The listing builds one solid part. Answer for the finished solid, in the listing's coordinates (mm). Face numbers are marked on the shaded views. Coordinates: 2 decimals unless noted, no trailing zeros. Order: outer loops, then holes, each group sorted by start corner. A loop starts at its lowest first (then second) coordinate and runs counter-clockwise, first axis right, second up.
from build123d import *

# Parameters (mm, degrees)
IZIM1_R                     = 8
IZIM1_R_2                   = 7
Y_KSEKLIK_EKSTR_ZYON1_DEPTH = 180
IZIM2_R                     = 1.5
KES_EKSTR_ZYON1_DEPTH       = 10


with BuildPart() as part:
    # Çizim1 → Yükseklik-Ekstrüzyon1 (new body)
    with BuildSketch(Plane(origin=(0, 0, 0), x_dir=(1, 0, 0), z_dir=(0, 1, 0))):
        with Locations(Location((0, 0, 0), (0, 0, 90))):
            Circle(IZIM1_R)
        with Locations(Location((0, 0, 0), (0, 0, 90))):
            Circle(IZIM1_R_2, mode=Mode.SUBTRACT)
    extrude(amount=Y_KSEKLIK_EKSTR_ZYON1_DEPTH)

    # Çizim2 → Kes-Ekstrüzyon1 (cut, symmetric)
    with BuildSketch(Plane.XY):
        with Locations((0, 11)):
            Circle(IZIM2_R)
        with Locations((0, 168)):
            Circle(IZIM2_R)
        with Locations((0, 158)):
            Circle(IZIM2_R)
        with Locations((0, 21)):
            Circle(IZIM2_R)
    extrude(amount=KES_EKSTR_ZYON1_DEPTH, both=True, mode=Mode.SUBTRACT)


solid = part.part
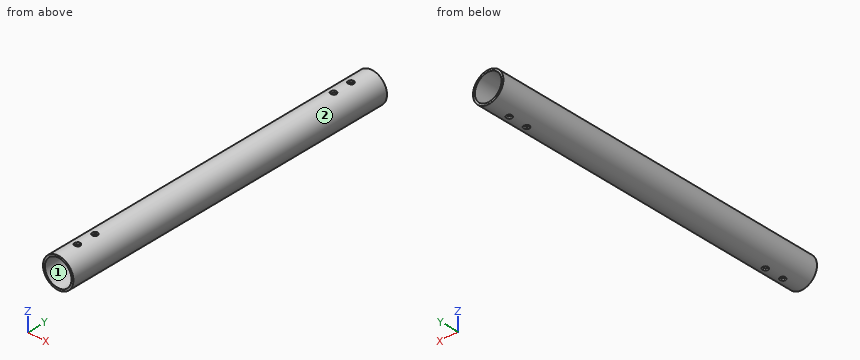
1) Section C-C (x = 0) is taken. Give the number of separate pieces and of enclosed holes in the cut face, then the cut area to 3 significant figures.
2) Determine the mould class of the marked faces 1 and 2 for opening direction X: released by +X, released by -X, zero draft, split by the parting line, or undercut.
3) Section D-D (y = 11) is taken. Give the vertices of the cut face in (x, z), then the cut area to 3 significant figures.
4) Section A-A (z = 0) is taken. Give the vertices of the cut face in (x, y).
5) Each of these flat-tipped pins is pushed along its axis until it touches: P1, Ø1.5, axis at x = -5.5, z = 3.5, coming from the +Y side; P2, Ø4, axis at x = 2.5, y = 107.5, coming from the +Z side; P3, Ø1, axis at y = 105.5, z = 4.5, coming from the +X side; P4, Ø3, axis at y = 99.5, z = -2.5, coming from the -X side. Where does it stop, or does it pass through?
6) Consider L1, parallel to Y at x = 0, z = 7.15; L2, parallel to Z at x = -0.5, y = 150; L3, parallel to X at y = 37, z = 0. Determine where each line is inside the solid, lowest interval first.
7) Section B-B (y = 41) is taken. Give the vertices of the cut face in (x, z), then the cut area to 3 significant figures.
Filled sheet:
1. separate pieces: 10
1. enclosed holes: 0
1. area: 336 mm2
2. face 1: undercut
2. face 2: split by the parting line
3. outline: (-1.5, -7.86) - (-1.5, -6.84) arc R7 cw to (-1.5, 6.84) - (-1.5, 7.86) arc R8 ccw to start; (1.5, -7.86) arc R8 ccw to (1.5, 7.86) - (1.5, 6.84) arc R7 cw to (1.5, -6.84) - close
3. area: 41.1 mm2
4. outline: (-8, 0) - (-7, 0) - (-7, 180) - (-8, 180) - close; (7, 0) - (8, 0) - (8, 180) - (7, 180) - close
5. P1: stops at y = 180
5. P2: stops at z = 7.98
5. P3: stops at x = 6.93
5. P4: stops at x = -7.94
6. L1: y = 0 to 9.5, 12.5 to 19.5, 22.5 to 156.5, 159.5 to 166.5, 169.5 to 180
6. L2: z = -7.98 to -6.98, 6.98 to 7.98
6. L3: x = -8 to -7, 7 to 8
7. outline: circle Ø16 at (0, 0); hole circle Ø14 at (0, 0)
7. area: 47.1 mm2
